Geometry check sheet. Reference: drawing and pictorial views, mm from the part's lowest x, y, z. A direction names the side the tool comes from. Round coordinates to 2 decimals unless told otherwise and drop trailing zeros. Write each loop counter-clockwise with the first axis right and the second up, starting at its lowest first coordinate (ties: lowest second). Pieces come first, ordered by that corner, then holes. Notation, with made-up numbers: (-31.5, 50) -> (-3.5, 50) arc R11 cw to (-3.5, 68) -> close; hole circle Ø6 at (-25, 11.25). An arc over 180 degrees is marked (long way). Answer as a JSON object with one key per item and string values. Group by question number.
(1) Sectioned sample at D-D on y = 44.5. Record the cut outline in (x, z) (1 decimal), and give its area (3 significant figures).
(2) Sectioned sample at A-A on x = 76.2. Record the cut outline in (y, z).
(3) Sectioned sample at B-B on z = 76.2. Record the cut outline in (x, y) (1 decimal).
(4) Scan lines: L1, parallel to X at y = 26, z = 76.2 (1 decimal); L2, parallel to Z at x = 76, y = 18. Record each from-to range of solid material in increasing order. Write a range as from..to.
(5) Sectioned sample at C-C on z = 50. Record the cut outline in (x, y) (1 decimal).
(6) Set-up check for the marked faces 1 and 2: record each of +Z, -Z, +X, -X, +Y, -Y from which the full face is reachable in a straight line by a thin tool's end or side.
(7) Gauge pin test, flat ends, axial feed: pin 1 Ø3 at (x, y) = (94, 42) entering from +Z; pin 2 Ø6 at (y, z) = (35.5, 48.5) entering from +X (1 decimal); pin 3 Ø4 at (x, y) = (103.5, 9) entering from +Z; pin 4 Ø5 at (x, z) = (7.78, 76.2) entering from +Y. Record the tip position at first contact, or that the pin passes through.
(8) Draft check along Z on the marked faces 3, 4 and 5. Enter one of: released by +Z, released by -Z, zero draft, split by the parting line, or undercut.
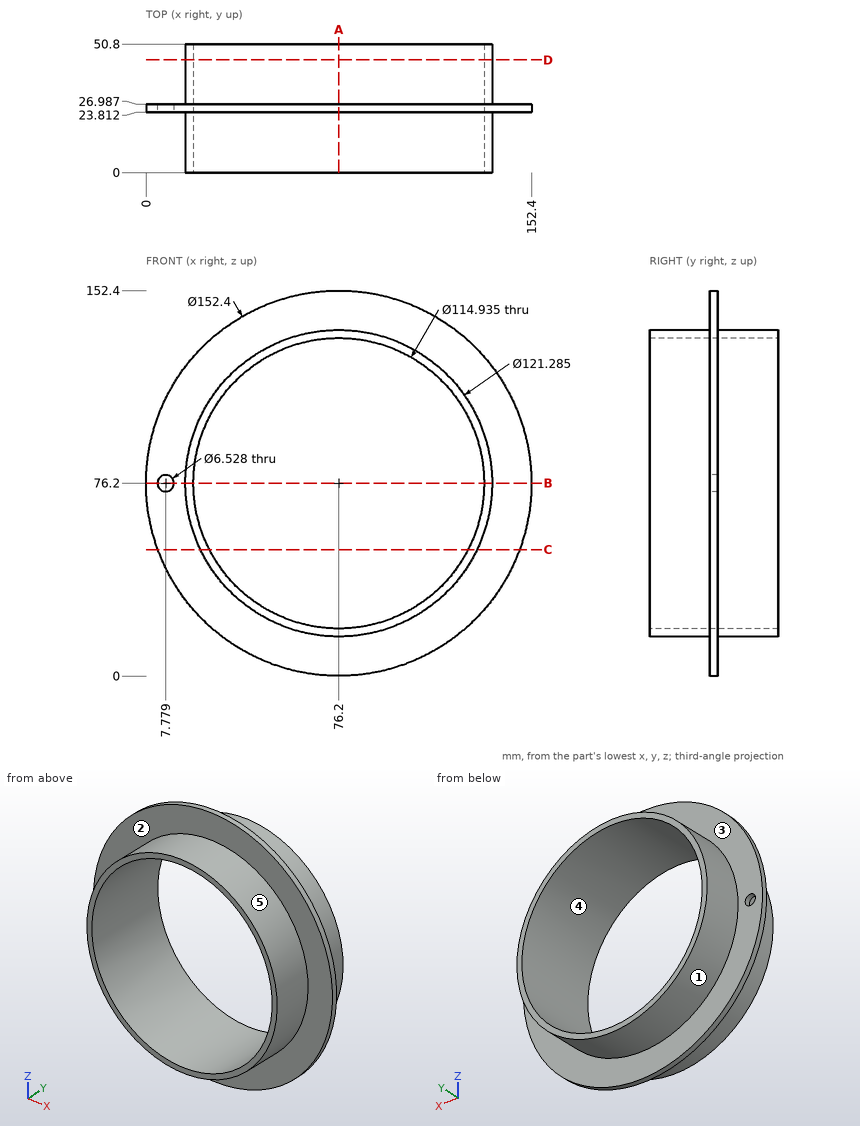
Computed values:
{
 "1": {"outline": "circle Ø121.3 at (76.2, 76.2); hole circle Ø114.9 at (76.2, 76.2)", "area": "1,180 mm2"},
 "2": {"outline": "(0, 15.56) -> (23.81, 15.56) -> (23.81, 0) -> (26.99, 0) -> (26.99, 15.56) -> (50.8, 15.56) -> (50.8, 18.73) -> (0, 18.73) -> close; (0, 133.67) -> (50.8, 133.67) -> (50.8, 136.84) -> (26.99, 136.84) -> (26.99, 152.4) -> (23.81, 152.4) -> (23.81, 136.84) -> (0, 136.84) -> close"},
 "3": {"outline": "(0, 23.8) -> (4.5, 23.8) -> (4.5, 27) -> (0, 27) -> close; (11, 23.8) -> (15.6, 23.8) -> (15.6, 0) -> (18.7, 0) -> (18.7, 50.8) -> (15.6, 50.8) -> (15.6, 27) -> (11, 27) -> close; (133.7, 0) -> (136.8, 0) -> (136.8, 23.8) -> (152.4, 23.8) -> (152.4, 27) -> (136.8, 27) -> (136.8, 50.8) -> (133.7, 50.8) -> close"},
 "4": {"L1": "0..4.5, 11..18.7, 133.7..152.4", "L2": "15.56..18.73, 133.67..136.84"},
 "5": {"outline": "(4.6, 23.8) -> (21.5, 23.8) -> (21.5, 0) -> (25.1, 0) -> (25.1, 50.8) -> (21.5, 50.8) -> (21.5, 27) -> (4.6, 27) -> close; (127.3, 0) -> (130.9, 0) -> (130.9, 23.8) -> (147.8, 23.8) -> (147.8, 27) -> (130.9, 27) -> (130.9, 50.8) -> (127.3, 50.8) -> close"},
 "6": {"face 1": "+Y", "face 2": "-Y"},
 "7": {"pin 1": "z = 134.61", "pin 2": "x = 131.6", "pin 3": "z = 131.31", "pin 4": "through"},
 "8": {"face 3": "zero draft", "face 4": "undercut", "face 5": "split by the parting line"}
}
